Work out the finished part from the listing and answer in its coordinate system (mm). Face numbers are marked on the shaded views. A direction names the side the tool comes from. Round coordinates to 2 decimals unless told otherwise and drop trailing zeros. Order: outer loops, then holes, each group sorted by start corner. A loop starts at its lowest first (then second) coordinate and runs counter-clockwise, first axis right, second up. Notation, with made-up numbers: M 65.25,-7.75 L 123.25,-7.75 A18 cw 123.25,-0.75 Z; hole C 35.5,13.5 d5. An arc over 180 degrees is marked long. Answer as a JSON object with one key per item and string values. Group by question number.
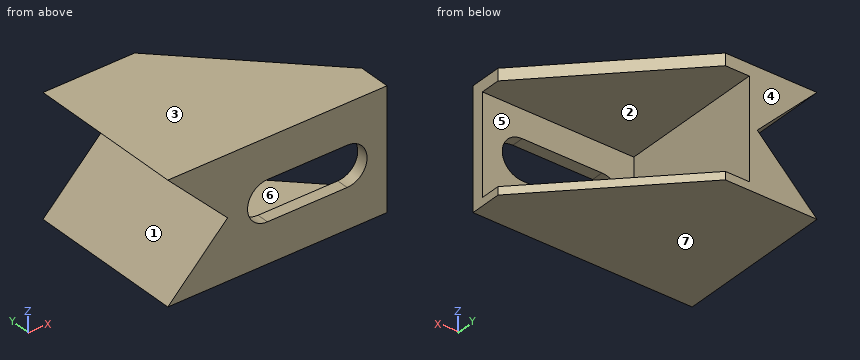
from build123d import *

# Parameters (mm, degrees)
BOSS_EXTRUDE1_DEPTH = 19.05
SHELL1_T            = -1.905
CUT_EXTRUDE1_DEPTH  = 1.905
BOSS_EXTRUDE2_DEPTH = 25.4
CUT_EXTRUDE2_START  = -23.495
SKETCH5_W           = 24.13
SKETCH5_H           = 15.875
CUT_EXTRUDE2_DEPTH  = 23.495


with BuildPart() as part:
    # Sketch1 → Boss-Extrude1 (new body)
    with BuildSketch(Plane.XY):
        Polygon((0, 0), (25.4, 0), (25.4, 5.08), (5.08, 25.4), (0, 25.4), align=None)
    extrude(amount=BOSS_EXTRUDE1_DEPTH)

    # Shell1
    shell1_openings = [part.faces().sort_by_distance(p)[0] for p in [
        (15.24, 15.24, 9.525),
    ]]
    offset(amount=SHELL1_T, openings=shell1_openings, kind=Kind.INTERSECTION)

    # Sketch2 → Cut-Extrude1 (cut)
    with BuildSketch(Plane.XZ):
        with BuildLine():
            Line((6.35, 12.7), (19.05, 12.7))
            ThreePointArc((19.05, 12.7), (22.225, 9.525), (19.05, 6.35))
            Line((19.05, 6.35), (6.35, 6.35))
            ThreePointArc((6.35, 6.35), (3.175, 9.525), (6.35, 12.7))
        make_face()
    extrude(amount=-CUT_EXTRUDE1_DEPTH, mode=Mode.SUBTRACT)

    # Sketch3 → Boss-Extrude2 (add)
    with BuildSketch(Plane(origin=(0, 25.4, 0), x_dir=(1, 0, 0), z_dir=(0, 1, 0))):
        Polygon((-9.525, 0), (0, -9.525), (0, 0), align=None)
        Polygon((0, -19.05), (0, -9.525), (-9.525, -19.05), align=None)
    extrude(amount=-BOSS_EXTRUDE2_DEPTH)

    # Sketch5 → Cut-Extrude2 (cut)
    with BuildSketch(Plane(origin=(0, 25.4, 0), x_dir=(1, 0, 0), z_dir=(0, 1, 0)).offset(CUT_EXTRUDE2_START)):
        with Locations((13.335, -9.2075)):
            Rectangle(SKETCH5_W, SKETCH5_H)
    extrude(amount=CUT_EXTRUDE2_DEPTH, mode=Mode.SUBTRACT)


solid = part.part
Item 1: Each of these flat-tipped pins is pushed along its axis until it touches: pin 1 (1.5 mm diameter, centred on y = 22, z = 9, fed in from -X) (3 decimals); pin 2 (8 mm diameter, centred on y = 8.5, z = 10.5, fed in from +X); pin 3 (5 mm diameter, centred on y = 22.5, z = 15, fed in from +X); pin 4 (3 mm diameter, centred on x = -3.5, z = 17, fed in from -Y). Where does it stop, or does it pass through?
Item 2: Consider L1, parallel to Z at x = 3.5, y = 2.5 (3 decimals); L2, parallel to Y at x = 5, z = 6 (3 decimals); L3, parallel to X at y = 24.5, z = 2 (3 decimals). Determine where each line is inside the solid, lowest interval first.
Item 3: Find section D-D (x = 15.5). Give the vertices of the cut face in (y, z) (3 decimals), and give its area (3 significant figures).
Item 4: A tool of negligible diameter and unlimited length cuts with its end or side. For the marked faces 1, 2 and 3, from which of +Z, -Z, +X, -X, +Y, -Y can it reach the whole face along a straight path? Write none if from no direction.
Item 5: Find section C-C (z = 17.75). Give the vertices of the cut face in (x, y) (3 decimals).
Item 6: The mould has two halves that part along Z. Classify the marked faces 4, 5, 6 and 7: +Z half, -Z half, draft (parallel to the pull), parting line (faces both ways), or undercut.
Item 7: Find section A-A (x = 11). Give the vertices of the cut face in (y, z) (3 decimals).
Item 8: Find section B-B (y = 16.5). Give the vertices of the cut face in (x, z) (3 decimals), and give its area (3 significant figures).
Responses:
{
 "1": {"pin 1": "stops at x = -1.275", "pin 2": "stops at x = 1.27", "pin 3": "stops at x = 9.26", "pin 4": "stops at y = 0"},
 "2": {"L1": "z = 0 to 1.27, 17.145 to 19.05", "L2": "y = 0 to 1.905", "L3": "x = -7.525 to 1.27"},
 "3": {"outline": "M 0,0 L 14.98,0 L 14.98,1.27 L 1.905,1.27 L 1.905,6.35 L 0,6.35 Z; M 0,12.7 L 1.905,12.7 L 1.905,17.145 L 14.98,17.145 L 14.98,19.05 L 0,19.05 Z", "area": "65.7 mm^2"},
 "4": {"face 1": "-X, +Y, -Y", "face 2": "+X, +Y", "face 3": "+Z, +X, -X, +Y, -Y"},
 "5": {"outline": "M -8.225,0 L 25.4,0 L 25.4,5.08 L 5.08,25.4 L -8.225,25.4 Z"},
 "6": {"face 4": "draft", "face 5": "undercut", "face 6": "undercut", "face 7": "-Z half"},
 "7": {"outline": "M 0,0 L 19.48,0 L 19.48,1.27 L 1.905,1.27 L 1.905,6.35 L 0,6.35 Z; M 0,12.7 L 1.905,12.7 L 1.905,17.145 L 19.48,17.145 L 19.48,19.05 L 0,19.05 Z"},
 "8": {"outline": "M -9.525,0 L 13.98,0 L 13.98,1.27 L 1.27,1.27 L 1.27,17.145 L 13.98,17.145 L 13.98,19.05 L -9.525,19.05 L 0,9.525 Z", "area": "155 mm^2"}
}
